from build123d import *

# Parameters (mm, degrees)
F0_W     = 9.75
F0_H     = 3
F0_W_2   = 3
F0_W_3   = 1.5
F1_DEPTH = 2
F2_W     = 4.5
F2_H     = 3
F3_DEPTH = 3.8
F4_R     = 1.65
F5_DEPTH = 9.001


with BuildPart() as f1:
    # F0 (on Front) → F1 (new body)
    with BuildSketch(Plane.XZ):
        Polygon((-8.25, 0), (0, 0), (0, 3), (-9.75, 3), (-9.75, 0), align=None)
        with Locations((4.875, 1.5)):
            Rectangle(F0_W, F0_H)
        Polygon((9.75, 3), (9.75, 0), (9.75, -3), (12.75, -3), (12.75, 3), align=None)
        with Locations((-11.25, 1.5)):
            Rectangle(F0_W_2, F0_H)
        with Locations((-11.25, -1.5)):
            Rectangle(F0_W_2, F0_H)
        Polygon((12.75, -3), (9.75, -3), (8.25, -3), (8.25, -6), (12.75, -6), align=None)
        with Locations((-11.25, -4.5)):
            Rectangle(F0_W_2, F0_H)
        with Locations((-9, -4.5)):
            Rectangle(F0_W_3, F0_H)
    extrude(amount=F1_DEPTH)

    # F2 (on face) → F3 (join)
    with BuildSketch(Plane.XZ.offset(2)):
        with Locations((-10.5, -4.5)):
            Rectangle(F2_W, F2_H)
        with Locations((10.5, -4.5)):
            Rectangle(F2_W, F2_H)
    extrude(amount=F3_DEPTH)

    # F4 (on face) → F5 (cut, through all)
    with BuildSketch(Plane(origin=(0, 0, -6), x_dir=(1, 0, 0), z_dir=(0, 0, -1))):
        with Locations((-10.5, 4)):
            Circle(F4_R)
        with Locations((10.5, 4)):
            Circle(F4_R)
    extrude(amount=-F5_DEPTH, mode=Mode.SUBTRACT)


solid = f1.part
Build history of the part. All positions in model axes, mm. A direction names the side the tool comes from. Give positions to 0.01 mm unless a question says otherwise; leave off trailing zeros. Order: outer loops, then holes, each group sorted by start corner. A loop starts at its lowest first (then second) coordinate and runs counter-clockwise, first axis right, second up. Notation, with made-up numbers: M 1.25,-23 L 52.25,-23 A26 cw 52.25,9 Z; hole C 78,89 d2. An arc over 180 degrees is marked long. Put each result on its own line as item: value.
Item 1: Cut at C-C on y = -4. Write the cut outline in (x, z), then the cut area to 3 significant figures.
Results are:
outline: M -12.75,-6 L -12.15,-6 L -12.15,-3 L -12.75,-3 Z; M -8.85,-6 L -8.25,-6 L -8.25,-3 L -8.85,-3 Z; M 8.25,-6 L 8.85,-6 L 8.85,-3 L 8.25,-3 Z; M 12.15,-6 L 12.75,-6 L 12.75,-3 L 12.15,-3 Z
area: 7.20 mm2
Item 2: Cut at D-D on z = -2. Write the cut outline in (x, y).
Results are:
outline: M -12.75,-2 L -9.75,-2 L -9.75,0 L -12.75,0 Z; M 9.75,-2 L 12.75,-2 L 12.75,0 L 9.75,0 Z
Item 3: Cut at A-A on z = -5. Write the cut outline in (x, y).
Results are:
outline: M -12.75,-5.8 L -8.25,-5.8 L -8.25,0 L -12.75,0 Z; M 8.25,-5.8 L 12.75,-5.8 L 12.75,0 L 8.25,0 Z; hole C -10.5,-4 d3.3; hole C 10.5,-4 d3.3
Item 4: Wall check: probe 1 along X at (y, z) = (-4, -5.4); probe 2 along Y at (x, z) = (-10.5, -3.6); probe 3 along X at (y, z) = (-1.8, -0.5). Give the ranges that are in metal, low to high.
Results are:
probe 1: -12.75 to -12.15, -8.85 to -8.25, 8.25 to 8.85, 12.15 to 12.75
probe 2: -5.8 to -5.65, -2.35 to 0
probe 3: -12.75 to -9.75, 9.75 to 12.75
Item 5: Which spindle directions (+Z, -Z, +X, -X, +Y, -Y) get a long thin tool onto all of the face, cutting with end or side? Do faces 4 (the face through (-10, -2.2, -3)), 5 (the face through (8.25, -3, -4)), 6 (the face through (-9.75, -1, -2)). Say none if no direction does.
Results are:
face 4: -Y
face 5: -Z, +Y, -Y
face 6: +Y, -Y
Item 6: Drop flat-ended pins along their axis: pin 1 Ø5 at (x, z) = (-1.5, -0.5) entering from -Y; pin 2 Ø1.3 at (x, y) = (-11, -3) entering from +Z; pin 3 Ø0.6 at (x, y) = (-4, -0.5) entering from -Z. Give the stop position or say it passes through.
Results are:
pin 1: y = -2
pin 2: z = -3
pin 3: z = 0
Item 7: Pull direction Z, two halves, no side cores. Call faces 1 (the face through (-11, -5.8, -4)), 2 (the face through (-11, -2, -6)), 3 (the face through (10, -2.2, -3)): +Z half, -Z half, draft (parallel to the pull), parting line (faces both ways), or undercut.
Results are:
face 1: draft
face 2: -Z half
face 3: undercut
Item 8: Cut at B-B on x = 10.5. Write the cut outline in (y, z), then the cut area to 3 significant figures.
Results are:
outline: M -5.8,-6 L -5.65,-6 L -5.65,-3 L -5.8,-3 Z; M -2.35,-6 L 0,-6 L 0,3 L -2,3 L -2,-3 L -2.35,-3 Z
area: 19.5 mm2
